Model file for the job. Use its own axes, mm. A direction names the side the tool comes from. Round coordinates to 2 decimals unless told otherwise and drop trailing zeros. Loops run counter-clockwise (first coordinate to the right, second up) from the corner with the lowest first, then second, coordinate; pieces in that order, holes last. Notation, with made-up numbers: M -35,74.5 L -8,74.5 A10 ccw -8,84.5 Z; hole C 35,-5 d9. An arc over 180 degrees is marked long. Use a Markdown table: item, result. Add a question column.
Q1. Tool access for faces 1 (the face through (-2.9, 0.1, 1.5)), 2 (the face through (2, 0, 0)), 3 (the face through (0, 0, 1)): list every direction of +Z, -Z, +X, -X, +Y, -Y with a clear straight run to the whole face (end or side of a thin tool).
Q2. Cut at B-B (z = 2). Give the cut face in (x, y).
Q3. Cut at A-A (z = 0.6). Give the cut face in (x, y), plus the area to 3 significant figures.
Q4. Mould opens along X. For faces 4 (the face through (3, 1, 0.75)), 5 (the face through (-0.867, -3.905, 0.37)), 6 (the face through (0, 1.45, 0.5)) say: +X half, -X half, draft (parallel to the pull), parting line (faces both ways), or undercut.
Q5. Pin check, flat tips, straight feed: pin 1 (1.4 mm diameter, centred on x = 0.5, y = 0.5, fed in from -Z); pin 2 (1.5 mm diameter, centred on x = -2, z = 1, fed in from -Y); pin 3 (0.5 mm diameter, centred on y = -0.5, z = 0.5, fed in from +X). Stop position of each tip, or through.
Q6. Probe line 1 (Y direction, x = 0, z = 2.45); line 2 (X direction, y = -1, z = 2.3); line 3 (Y direction, x = 1, z = 0.55). List the from-to ranges inside material, lowest first. Write a range as from..to.
Q7. Cut at C-C (x = 3). Give the cut face in (y, z), plus the area to 3 significant figures.
from build123d import *

# Parameters (mm, degrees)
SZKIC1_R                    = 4
DODANIE_WYCI_GNI_CIE1_DEPTH = 0.75
SZKIC2_R                    = 2.9
DODANIE_WYCI_GNI_CIE2_DEPTH = 2.5
SZKIC3_W                    = 2.5
SZKIC3_H                    = 2.5
WYTNIJ_WYCI_GNI_CIE1_DEPTH  = 1
ZAOKR_GLENIE2_R             = 1
SZKIC4_W                    = 2.9
SZKIC4_H                    = 2.9
WYTNIJ_WYCI_GNI_CIE2_DEPTH  = 1
WYTNIJ_WYCI_GNI_CIE3_DEPTH  = 1
WYTNIJ_WYCI_GNI_CIE4_DEPTH  = 0.75


with BuildPart() as part:
    # Szkic1 → Dodanie-wyciągnięcie1 (new body)
    with BuildSketch(Plane.XY):
        Circle(SZKIC1_R)
    extrude(amount=DODANIE_WYCI_GNI_CIE1_DEPTH)

    # Szkic2 → Dodanie-wyciągnięcie2 (add)
    with BuildSketch(Plane.XY.offset(0.75)):
        Circle(SZKIC2_R)
    extrude(amount=DODANIE_WYCI_GNI_CIE2_DEPTH)

    # Szkic3 → Wytnij-wyciągnięcie1 (cut)
    with BuildSketch(Plane(origin=(0, 0, 0), x_dir=(-1, 0, 0), z_dir=(0, 0, -1))):
        Rectangle(SZKIC3_W, SZKIC3_H)
    extrude(amount=-WYTNIJ_WYCI_GNI_CIE1_DEPTH, mode=Mode.SUBTRACT)

    # Zaokrąglenie2
    zaokr_glenie2_edges = [part.edges().sort_by_distance(p)[0] for p in [
        (-2.9, 0, 3.25),
    ]]
    fillet(zaokr_glenie2_edges, radius=ZAOKR_GLENIE2_R)

    # Szkic4 → Wytnij-wyciągnięcie2 (cut)
    with BuildSketch(Plane(origin=(0, 0, 0), x_dir=(-1, 0, 0), z_dir=(0, 0, -1))):
        Rectangle(SZKIC4_W, SZKIC4_H)
    extrude(amount=-WYTNIJ_WYCI_GNI_CIE2_DEPTH, mode=Mode.SUBTRACT)

    # Szkic5 → Wytnij-wyciągnięcie3 (cut)
    with BuildSketch(Plane.XY.offset(3.25)):
        with BuildLine():
            Line((-0.921182905, 1.584423241), (-0.293779059, 1.584423241))
            add(Edge.make_bspline(
                [(-0.293779059, 1.584423241), (-0.252307855, 1.584276042), (-0.17254705, 1.583992937), (-0.057536324, 1.579526289), (0.048116843, 1.573310581), (0.144568883, 1.563825246), (0.23177853, 1.551248838), (0.309833189, 1.536423335), (0.378730579, 1.519526495), (0.439051754, 1.4984717), (0.493488632, 1.47472221), (0.54423137, 1.44743361), (0.592399429, 1.416909768), (0.637670857, 1.382347519), (0.680439074, 1.344368629), (0.720784764, 1.302934869), (0.758137806, 1.257694897), (0.792266907, 1.208934573), (0.823372836, 1.15763983), (0.850863953, 1.10374024), (0.873219776, 1.04719832), (0.892973541, 0.988831223), (0.907201538, 0.927804579), (0.917096902, 0.864712494), (0.924341901, 0.799332876), (0.924758453, 0.754916866), (0.924970941, 0.73225978)],
                knots=[0, 0, 0, 0, 1.749336639, 3.364467119, 4.854658419, 6.213483162, 7.451590619, 8.570285859, 9.5643256, 10.440900261, 11.26203566, 12.067320669, 12.869050712, 13.665104639, 14.467235401, 15.27997916, 16.102287765, 16.939272006, 17.78853747, 18.631303466, 19.488103222, 20.351255419, 21.228522269, 22.127379805, 23.044756219, 24, 24, 24, 24], degree=3))
            add(Edge.make_bspline(
                [(0.924970941, 0.73225978), (0.924418974, 0.708610987), (0.923336666, 0.662240014), (0.917506767, 0.594124836), (0.906851544, 0.528956999), (0.890712658, 0.466927305), (0.872163104, 0.407263723), (0.847496956, 0.351067083), (0.819658771, 0.297520087), (0.786596171, 0.247380176), (0.750311583, 0.199533643), (0.70811337, 0.155813667), (0.662735328, 0.113870465), (0.611626594, 0.076331215), (0.557040086, 0.040657651), (0.497891228, 0.008327901), (0.434566047, -0.021470729), (0.390045308, -0.038088504), (0.367278634, -0.046586374)],
                knots=[0, 0, 0, 0, 1.099860209, 2.156625411, 3.176576793, 4.16617041, 5.135385252, 6.078461593, 7.016046972, 7.938469504, 8.868247731, 9.803980173, 10.76021508, 11.73834243, 12.748633912, 13.790971185, 14.870363756, 16, 16, 16, 16], degree=3))
            Line((0.367278634, -0.046586374), (1.059586326, -1.415576759))
            Line((1.059586326, -1.415576759), (0.461028634, -1.415576759))
            Line((0.461028634, -1.415576759), (-0.200029059, -0.107884451))
            Line((-0.200029059, -0.107884451), (-0.382721366, -0.107884451))
            Line((-0.382721366, -0.107884451), (-0.382721366, -1.415576759))
            Line((-0.382721366, -1.415576759), (-0.921182905, -1.415576759))
            Line((-0.921182905, -1.415576759), (-0.921182905, 1.584423241))
        make_face()
        with BuildLine():
            Line((-0.382721366, 0.430577087), (-0.172985789, 0.430577087))
            add(Edge.make_bspline(
                [(-0.172985789, 0.430577087), (-0.147343872, 0.430865884), (-0.098245109, 0.431418867), (-0.02763464, 0.433983833), (0.036496506, 0.440164132), (0.09442373, 0.44797271), (0.146438515, 0.456988841), (0.192076908, 0.469909503), (0.232042127, 0.48375432), (0.265860584, 0.500959836), (0.294754296, 0.520526239), (0.319702167, 0.54275416), (0.340337634, 0.568480148), (0.357321675, 0.597005082), (0.370533413, 0.628581257), (0.38017697, 0.66286204), (0.385566291, 0.700237931), (0.386186351, 0.726032386), (0.386509403, 0.739471318)],
                knots=[0, 0, 0, 0, 1.688639943, 3.233382647, 4.650958383, 5.928841754, 7.082724185, 8.122798841, 9.049171256, 9.863274652, 10.613301712, 11.341792392, 12.054588806, 12.776240173, 13.521029143, 14.301969904, 15.115324896, 16, 16, 16, 16], degree=3))
            add(Edge.make_bspline(
                [(0.386509403, 0.739471318), (0.385898644, 0.755370556), (0.384698922, 0.786601663), (0.372793947, 0.831563506), (0.353843798, 0.873178768), (0.327868335, 0.911259421), (0.295155616, 0.94464355), (0.257615189, 0.974071926), (0.214436843, 0.997341683), (0.174456944, 1.012690168), (0.138084581, 1.021873324), (0.10525967, 1.028716531), (0.067248226, 1.033566508), (0.024021552, 1.038710772), (-0.024310165, 1.042046567), (-0.078010364, 1.044481033), (-0.136924816, 1.045477092), (-0.177993785, 1.045795515), (-0.199428097, 1.045961703)],
                knots=[0, 0, 0, 0, 1.020303359, 2.004196876, 2.966617323, 3.9489082, 4.950758222, 5.960522915, 7.003732012, 8.091992268, 8.70421221, 9.413913587, 10.24622431, 11.166358409, 12.212345909, 13.359657661, 14.621978493, 16, 16, 16, 16], degree=3))
            Line((-0.199428097, 1.045961703), (-0.382721366, 1.045961703))
            Line((-0.382721366, 1.045961703), (-0.382721366, 0.430577087))
        make_face(mode=Mode.SUBTRACT)
    extrude(amount=-WYTNIJ_WYCI_GNI_CIE3_DEPTH, mode=Mode.SUBTRACT)

    # Szkic6 → Wytnij-wyciągnięcie4 (cut)
    with BuildSketch(Plane.XY.offset(3.25)):
        with BuildLine():
            Line((-0.199428097, 1.045961703), (-0.382721366, 1.045961703))
            Line((-0.382721366, 1.045961703), (-0.382721366, 0.430577087))
            Line((-0.382721366, 0.430577087), (-0.172985789, 0.430577087))
            add(Edge.make_bspline(
                [(-0.172985789, 0.430577087), (-0.147343872, 0.430865884), (-0.098245109, 0.431418867), (-0.02763464, 0.433983833), (0.036496506, 0.440164132), (0.09442373, 0.44797271), (0.146438515, 0.456988841), (0.192076908, 0.469909503), (0.232042127, 0.48375432), (0.265860584, 0.500959836), (0.294754296, 0.520526239), (0.319702167, 0.54275416), (0.340337634, 0.568480148), (0.357321675, 0.597005082), (0.370533413, 0.628581257), (0.38017697, 0.66286204), (0.385566291, 0.700237931), (0.386186351, 0.726032386), (0.386509403, 0.739471318)],
                knots=[0, 0, 0, 0, 0.105539996, 0.202086415, 0.290684899, 0.37055261, 0.442670262, 0.507674928, 0.565573203, 0.616454666, 0.663331357, 0.708862024, 0.7534118, 0.798515011, 0.845064321, 0.893873119, 0.944707806, 1, 1, 1, 1], degree=3))
            add(Edge.make_bspline(
                [(0.386509403, 0.739471318), (0.385898644, 0.755370556), (0.384698922, 0.786601663), (0.372793947, 0.831563506), (0.353843798, 0.873178768), (0.327868335, 0.911259421), (0.295155616, 0.94464355), (0.257615189, 0.974071926), (0.214436843, 0.997341683), (0.174456944, 1.012690168), (0.138084581, 1.021873324), (0.10525967, 1.028716531), (0.067248226, 1.033566508), (0.024021552, 1.038710772), (-0.024310165, 1.042046567), (-0.078010364, 1.044481033), (-0.136924816, 1.045477092), (-0.177993785, 1.045795515), (-0.199428097, 1.045961703)],
                knots=[0, 0, 0, 0, 0.06376896, 0.125262305, 0.185413583, 0.246806762, 0.309422389, 0.372532682, 0.437733251, 0.505749517, 0.544013263, 0.588369599, 0.640389019, 0.697897401, 0.763271619, 0.834978604, 0.913873656, 1, 1, 1, 1], degree=3))
        make_face()
    extrude(amount=-WYTNIJ_WYCI_GNI_CIE4_DEPTH, mode=Mode.SUBTRACT)


solid = part.part
Checked values:
| question | item | result |
|---|---|---|
| 1 | face 1 | +Z |
| 1 | face 2 | -Z, +X, -X, +Y, -Y |
| 1 | face 3 | -Z |
| 2 | outline | C 0,0 d5.8 |
| 3 | outline | C 0,0 d8; hole M -1.45,-1.45 L 1.45,-1.45 L 1.45,1.45 L -1.45,1.45 Z |
| 3 | area | 41.9 mm^2 |
| 4 | face 4 | draft |
| 4 | face 5 | parting line |
| 4 | face 6 | undercut |
| 5 | pin 1 | stops at z = 1 |
| 5 | pin 2 | stops at y = -3.79 |
| 5 | pin 3 | stops at x = 3.99 |
| 6 | line 1 | y = -2.88..-0.5, 0.44..1.04, 1.58..2.88 |
| 6 | line 2 | x = -2.72..-0.92, -0.38..0.25, 0.85..2.72 |
| 6 | line 3 | y = -3.87..-1.45, 1.45..3.87 |
| 7 | outline | M -2.65,0 L 2.65,0 L 2.65,0.75 L -2.65,0.75 Z |
| 7 | area | 3.97 mm^2 |
